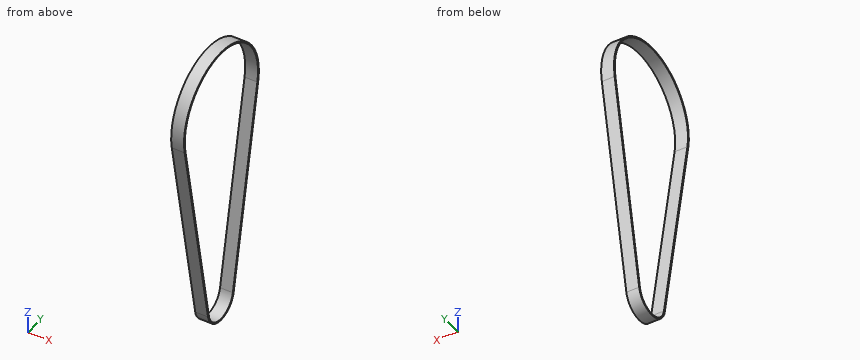
Autodesk Inventor part; units mm, degrees
ref_plane "YZ Plane" through (0, 0, 0) normal (1, 0, 0) x (0, 1, 0)
ref_plane "XZ Plane" through (0, 0, 0) normal (0, 1, 0) x (-1, 0, 0)
ref_plane "XY Plane" through (0, 0, 0) normal (0, 0, 1) x (1, 0, 0)
sketch "スケッチ1" plane through (0, 0, 0) normal (1, 0, 0) x (0, 1, 0)
  arc A0 (45.1681, -8.7086) -> (-45.2398, -8.3282) centre (0, 0) ccw
  arc A1 (-16.4172, -164.8953) -> (15.029, -165.0277) centre (-0.6816, -161.9986) ccw
  line L0 (45.1681, -8.7086) -> (15.029, -165.0277)
  line L1 (-45.2398, -8.3282) -> (-16.4172, -164.8953)
  arc A2 (44.1862, -8.5193) -> (-44.2563, -8.1472) centre (0, 0) ccw
  arc A3 (-15.4338, -164.7143) -> (14.0471, -164.8383) centre (-0.6816, -161.9986) ccw
  line L2 (44.1862, -8.5193) -> (14.0471, -164.8383)
  line L3 (-44.2563, -8.1472) -> (-15.4338, -164.7143)
  dimension "d0" = 92
  dimension "d1" = 32
  dimension "d2" = 100
  dimension "d3" = 90
  dimension "d4" = 30
extrude "押し出し1" add sketch "スケッチ1" along normal blind 10
properties part number "type4" material "ゴム"
Can you work these out from the model? Positions are in its coordinate system, mm. Coordinates: 2 decimals unless noted, no trailing zeros. Loops run counter-clockwise (first coordinate to the right, second up) from the corner with the lowest first, then second, coordinate; pieces in that order, holes last.
1) For pin 1 (5 mm diameter, centred on x = 7.5, z = 15.5, fed in from -Y); pin 2 (6 mm diameter, centred on x = 6, y = 14.5, fed in from -Z); pin 3 (4 mm diameter, centred on x = 4, z = -68.5, fed in from -Y), each with a flat end and sliding along its axis, tell me the tip position at first contact or that it passes through.
2) Imagine slicing it at C-C on y = 26. List the corners of the cut face in (x, z) for me.
3) Imagine slicing it at A-A on x = 7. List the corners of the cut face in (y, z) for me, plus the area to 3 significant figures.
4) Imagine slicing it at B-B on z = 10.5. List the corners of the cut face in (x, y) for me, plus the area to 3 significant figures.
5) I need wall thicknesses on probe 1 along Y at (x, z) = (5, 4); probe 2 along Y at (x, z) = (7, -48.5); probe 3 along Z at (x, y) = (5, -8.5). Which ranges of each line are inside material? Lowest first, please.
Completed:
1. pin 1: stops at y = -44.12
1. pin 2: stops at z = -172.37
1. pin 3: stops at y = -34.53
2. outline: (0, -108.13) - (10, -108.13) - (10, -102.84) - (0, -102.84) - close; (0, 36.73) - (10, 36.73) - (10, 37.95) - (0, 37.95) - close
3. outline: (-45.24, -8.33) - (-16.42, -164.9) arc R16 ccw to (15.03, -165.03) - (45.17, -8.71) arc R46 ccw (long way) to start; hole (-44.26, -8.15) - (-15.43, -164.71) arc R15 ccw to (14.05, -164.84) - (44.19, -8.52) arc R45 ccw (long way) to start
3. area: 521 mm2
4. outline: (0, -44.79) - (10, -44.79) - (10, -43.76) - (0, -43.76) - close; (0, 43.76) - (10, 43.76) - (10, 44.79) - (0, 44.79) - close
4. area: 20.6 mm2
5. probe 1: y = -45.83 to -44.82, 44.82 to 45.83
5. probe 2: y = -37.84 to -36.83, 36.48 to 37.5
5. probe 3: z = -175.96 to -174.8, 44.19 to 45.21
